```python
from build123d import *

# Parameters (mm, degrees)
F2_W     = 291
F2_H     = 147
F3_DEPTH = 5
F5_D     = 5.5
F6_R     = 3
F7_DEPTH = 5.001


# Not quite as in the source:
# - a pattern or mirror of a feature is missing from the dataset's text; its kind, count and spacing are read off the source's solid


with BuildPart() as f3:
    # F2 (on Top) → F3 (new body)
    with BuildSketch(Plane.XY):
        Rectangle(F2_W, F2_H)
        with BuildLine():
            ThreePointArc((-72, -13.5), (-85.5, 0), (-72, 13.5))
            Line((-72, 13.5), (72, 13.5))
            ThreePointArc((72, 13.5), (85.5, 0), (72, -13.5))
            Line((72, -13.5), (-72, -13.5))
        make_face(mode=Mode.SUBTRACT)
    extrude(amount=-F3_DEPTH)

    # F5 (through all)
    with Locations(Plane.XY):
        with Locations((-120, -50)):
            f5 = Hole(F5_D / 2)

    # F5_copies: F5 across plane
    add(f5.mirror(Plane(origin=(0, 0, 0), x_dir=(0, 0, 1), z_dir=(1, 0, 0))), mode=Mode.SUBTRACT)

    # F5_copies1: F5 across plane
    add(f5.mirror(Plane.ZX), mode=Mode.SUBTRACT)

    # F5_copies2: F5 across plane
    add(f5.mirror(Plane(origin=(0, 0, 0), x_dir=(-0.3846153846, 0.9230769231, 0), z_dir=(0.9230769231, 0.3846153846, 0))), mode=Mode.SUBTRACT)

    # F6 (on Top) → F7 (cut, through all)
    with BuildSketch(Plane.XY):
        with Locations((-137.5, -14)):
            Circle(F6_R)
    f7 = extrude(amount=-F7_DEPTH, mode=Mode.SUBTRACT)

    # F7_copies: F7 across plane
    add(f7.mirror(Plane(origin=(0, 0, 0), x_dir=(0, 0, 1), z_dir=(1, 0, 0))), mode=Mode.SUBTRACT)

    # F7_copies1: F7 across plane
    add(f7.mirror(Plane.ZX), mode=Mode.SUBTRACT)

    # F7_copies2: F7 across plane
    add(f7.mirror(Plane(origin=(0, 0, 0), x_dir=(-0.1012944786, 0.9948564864, 0), z_dir=(0.9948564864, 0.1012944786, 0))), mode=Mode.SUBTRACT)


solid = f3.part
```
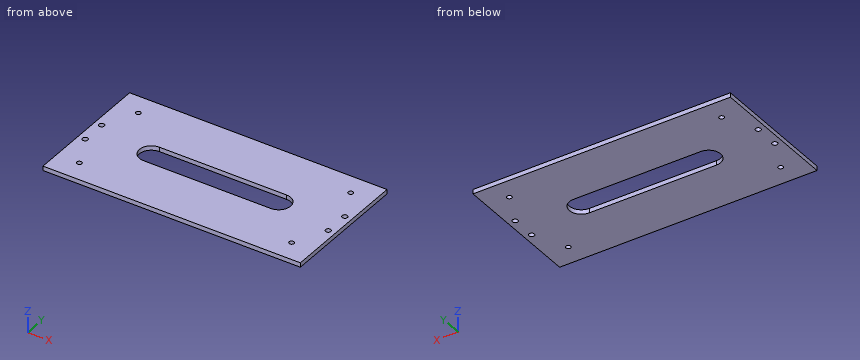
Part model, mm, in its own coordinate system. Round coordinates to 2 decimals unless told otherwise and drop trailing zeros. Write each loop counter-clockwise with the first axis right and the second up, starting at its lowest first coordinate (ties: lowest second). Pieces come first, ordered by that corner, then holes.
Item 1: Cut at C-C, the plane y = -8. Give the cut face in (x, z).
Results:
outline: (-145.5, -5) - (-82.87, -5) - (-82.87, 0) - (-145.5, 0) - close; (82.87, -5) - (145.5, -5) - (145.5, 0) - (82.87, 0) - close
Item 2: Cut at B-B, the plane x = -52.5. Give the cut face in (y, z), plus the area to 3 significant figures.
Results:
outline: (-73.5, -5) - (-13.5, -5) - (-13.5, 0) - (-73.5, 0) - close; (13.5, -5) - (73.5, -5) - (73.5, 0) - (13.5, 0) - close
area: 600 mm2
Item 3: Cut at A-A, the plane y = -50. Give the cut face in (x, z).
Results:
outline: (-145.5, -5) - (-122.75, -5) - (-122.75, 0) - (-145.5, 0) - close; (-117.25, -5) - (117.25, -5) - (117.25, 0) - (-117.25, 0) - close; (122.75, -5) - (145.5, -5) - (145.5, 0) - (122.75, 0) - close
Item 4: Probe L1, parallel to Y at x = 137.5, z = -2.2; L2, parallel to Y at x = 120, z = -1.7; L3, parallel to Y at x = -59.5, z = -1.75. List the from-to ranges inside material, lowest first.
Results:
L1: y = -73.5 to -17, -11 to 11, 17 to 73.5
L2: y = -73.5 to -52.75, -47.25 to 47.25, 52.75 to 73.5
L3: y = -73.5 to -13.5, 13.5 to 73.5
